```python
from build123d import *

# Parameters (mm, degrees)
SKETCH1_W             = 50
SKETCH1_H             = 60
BOSS_EXTRUDE1_DEPTH   = 3
CAVITY8_START         = -10
CAVITY8_OUTLINE_W     = 3
CAVITY8_OUTLINE_H     = 3
CAVITY8_DEPTH         = 20
CAVITY8_START_2       = -30
CAVITY8_2_OUTLINE_W   = 10
CAVITY8_2_OUTLINE_H   = 3
CAVITY8_2_OUTLINE_W_2 = 3
CAVITY8_2_DEPTH       = 3
CAVITY8_START_3       = 27
CAVITY8_3_OUTLINE_W   = 10
CAVITY8_3_OUTLINE_H   = 3
CAVITY8_3_OUTLINE_W_2 = 3
CAVITY8_3_DEPTH       = 3
CAVITY8_START_4       = -27
CAVITY8_4_OUTLINE_W   = 3
CAVITY8_4_OUTLINE_H   = 3
CAVITY8_4_DEPTH       = 7
CAVITY8_START_5       = 20
CAVITY8_5_OUTLINE_W   = 3
CAVITY8_5_OUTLINE_H   = 3
CAVITY8_5_DEPTH       = 7


# Read off the part's stored shape, not the designer's step: Cavity8
with BuildPart() as part:
    # Sketch1 → Boss-Extrude1 (new body)
    with BuildSketch(Plane.XY):
        Rectangle(SKETCH1_W, SKETCH1_H)
    extrude(amount=BOSS_EXTRUDE1_DEPTH)

    # Cavity8 outline → Cavity8 (cut)
    with BuildSketch(Plane(origin=(0, 0, 0), x_dir=(1, 0, 0), z_dir=(0, 1, 0)).offset(CAVITY8_START)):
        with Locations((23.5, -1.5)):
            Rectangle(CAVITY8_OUTLINE_W, CAVITY8_OUTLINE_H)
        with Locations((-23.5, -1.5)):
            Rectangle(CAVITY8_OUTLINE_W, CAVITY8_OUTLINE_H)
    extrude(amount=CAVITY8_DEPTH, mode=Mode.SUBTRACT)

    # Cavity8 2 outline → Cavity8 2 (cut)
    with BuildSketch(Plane(origin=(0, 0, 0), x_dir=(1, 0, 0), z_dir=(0, 1, 0)).offset(CAVITY8_START_2)):
        with Locations((10, -1.5)):
            Rectangle(CAVITY8_2_OUTLINE_W, CAVITY8_2_OUTLINE_H)
        with Locations((-10, -1.5)):
            Rectangle(CAVITY8_2_OUTLINE_W, CAVITY8_2_OUTLINE_H)
        with Locations((23.5, -1.5)):
            Rectangle(CAVITY8_2_OUTLINE_W_2, CAVITY8_2_OUTLINE_H)
        with Locations((-23.5, -1.5)):
            Rectangle(CAVITY8_2_OUTLINE_W_2, CAVITY8_2_OUTLINE_H)
    extrude(amount=CAVITY8_2_DEPTH, mode=Mode.SUBTRACT)

    # Cavity8 3 outline → Cavity8 3 (cut)
    with BuildSketch(Plane(origin=(0, 0, 0), x_dir=(1, 0, 0), z_dir=(0, 1, 0)).offset(CAVITY8_START_3)):
        with Locations((10, -1.5)):
            Rectangle(CAVITY8_3_OUTLINE_W, CAVITY8_3_OUTLINE_H)
        with Locations((-10, -1.5)):
            Rectangle(CAVITY8_3_OUTLINE_W, CAVITY8_3_OUTLINE_H)
        with Locations((23.5, -1.5)):
            Rectangle(CAVITY8_3_OUTLINE_W_2, CAVITY8_3_OUTLINE_H)
        with Locations((-23.5, -1.5)):
            Rectangle(CAVITY8_3_OUTLINE_W_2, CAVITY8_3_OUTLINE_H)
    extrude(amount=CAVITY8_3_DEPTH, mode=Mode.SUBTRACT)

    # Cavity8 4 outline → Cavity8 4 (cut)
    with BuildSketch(Plane(origin=(0, 0, 0), x_dir=(1, 0, 0), z_dir=(0, 1, 0)).offset(CAVITY8_START_4)):
        with Locations((23.5, -1.5)):
            Rectangle(CAVITY8_4_OUTLINE_W, CAVITY8_4_OUTLINE_H)
        with Locations((-23.5, -1.5)):
            Rectangle(CAVITY8_4_OUTLINE_W, CAVITY8_4_OUTLINE_H)
    extrude(amount=CAVITY8_4_DEPTH, mode=Mode.SUBTRACT)

    # Cavity8 5 outline → Cavity8 5 (cut)
    with BuildSketch(Plane(origin=(0, 0, 0), x_dir=(1, 0, 0), z_dir=(0, 1, 0)).offset(CAVITY8_START_5)):
        with Locations((23.5, -1.5)):
            Rectangle(CAVITY8_5_OUTLINE_W, CAVITY8_5_OUTLINE_H)
        with Locations((-23.5, -1.5)):
            Rectangle(CAVITY8_5_OUTLINE_W, CAVITY8_5_OUTLINE_H)
    extrude(amount=CAVITY8_5_DEPTH, mode=Mode.SUBTRACT)


solid = part.part
```
The listing builds one solid part. Answer for the finished solid, in the listing's coordinates (mm). A direction names the side the tool comes from. Coordinates: 2 decimals unless noted, no trailing zeros. Write each loop counter-clockwise with the first axis right and the second up, starting at its lowest first coordinate (ties: lowest second). Pieces come first, ordered by that corner, then holes. Notation, with made-up numbers: (59.25, 14.5) - (69.25, 14.5) arc R25 ccw to (69.25, 43.5) - close; hole circle Ø7 at (26.25, 69.5). An arc over 180 degrees is marked (long way). One line per item, written item: value.
1) Find section A-A (y = 24.5). Give the vertices of the cut face in (x, z), and give its area (3 significant figures).
Geometry check:
outline: (-22, 0) - (22, 0) - (22, 3) - (-22, 3) - close
area: 132 mm2
2) Each of these flat-tipped pins is pushed along its axis until it touches: pin 1 Ø1.5 at (y, z) = (-29, 1.5) entering from -X; pin 2 Ø6 at (x, y) = (6.5, 4.5) entering from -Z; pin 3 Ø0.9 at (x, z) = (-9.5, 2) entering from +Y; pin 4 Ø1.5 at (x, z) = (-23.5, 1) entering from -Y. Where does it stop, or does it pass through?
Geometry check:
pin 1: stops at x = -22
pin 2: stops at z = 0
pin 3: stops at y = 27
pin 4: stops at y = -20
3) A tool of negligible diameter and unlimited length cuts with its end or side. For faces 4 (the flat face through (15, -29, 2)), 5 (the flat face through (-5, 28, 2)), 6 (the flat face through (-24, -20, 1)), from which of +Z, -Z, +X, -X, +Y, -Y can it reach the whole face along a straight path? Write none if from no direction.
Geometry check:
face 4: +Z, -Z, -Y
face 5: +Z, -Z, +Y
face 6: +Z, -Z, -X, -Y
4) Consider line 1 along Y through (x, z) = (9.5, 1.6); line 2 along X through (y, z) = (25, 0.4). Determine where each line is inside the solid, lowest interval first. Write a range as from..to.
Geometry check:
line 1: y = -27..27
line 2: x = -22..22
5) Find section B-B (x = -11.5). Give the vertices of the cut face in (y, z), and give its area (3 significant figures).
Geometry check:
outline: (-27, 0) - (27, 0) - (27, 3) - (-27, 3) - close
area: 162 mm2
6) For a pull along X with two mould halves and no side action, classify faces 1 (the flat face through (23, -10, 1)), 2 (the flat face through (-22, 25, 2)), 3 (the flat face through (5, 28, 2)) as pulls with the +X half, pulls with the -X half, needs draft (parallel to the pull), parting line crosses it, or undercut.
Geometry check:
face 1: needs draft
face 2: pulls with the -X half
face 3: undercut
